CAD build for the part. Positions are in the model's coordinates, mm. Give positions to 0.01 mm unless a question says otherwise; leave off trailing zeros. Order: outer loops, then holes, each group sorted by start corner. A loop starts at its lowest first (then second) coordinate and runs counter-clockwise, first axis right, second up. Notation, with made-up numbers: (67.5, 81.5) -> (105.5, 81.5) arc R35 ccw to (105.5, 120.5) -> close; hole circle Ø3 at (85, 3.5). An arc over 180 degrees is marked (long way). Use one line per item in the form item = value. Start each with the question number.
1) Drop flat-ended pins along their axis: P1, Ø2, axis at y = 2, z = -4.5, coming from the +X side; P2, Ø1.5, axis at y = 8.5, z = 3, coming from the +X side; P3, Ø1.5, axis at x = 2, z = 7.5, coming from the -Y side. Give the stop position or say it passes through.
2) Cut at A-A, the plane x = 1. Give the cut face in (y, z), and give its area (3 significant figures).
3) Probe line 1 (X direction, y = -8.25, z = -1); line 2 (Y direction, x = 2.5, z = -7); line 3 (Y direction, x = 2, z = 4.75). List the from-to ranges inside material, lowest first.
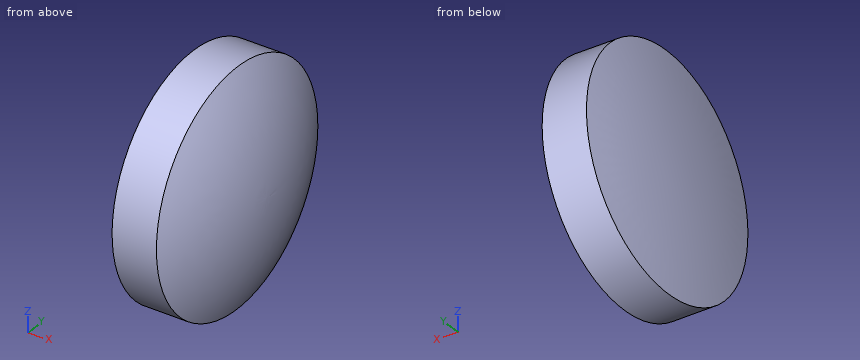
from build123d import *

# Parameters (mm, degrees)
F0_R     = 13.25
F1_DEPTH = 5


with BuildPart() as f1:
    # F0 (on Right) → F1 (new body)
    with BuildSketch(Plane.YZ):
        Circle(F0_R)
    extrude(amount=F1_DEPTH)

    # F2 (on Top) → F4 (revolve)
    with BuildSketch(Plane.XY):
        with BuildLine():
            ThreePointArc((8.325502, 0), (7.481431, 6.830473), (5, 13.25))
            Line((5, 13.25), (5, 0))
            Line((5, 0), (8.325502, 0))
        make_face()
    revolve(axis=Axis((5.30408, 0, 0), (1, 0, 0)))

    # F5 (on Front) → F6 (revolve)
    with BuildSketch(Plane.XZ):
        with BuildLine():
            Line((-1.236098, 0), (0, 0))
            Line((0, 0), (0, 13.25))
            ThreePointArc((0, 13.25), (-0.926404, 6.653767), (-1.236098, 0))
        make_face()
    revolve(axis=Axis((-0.618049, 0, 0), (-1, 0, 0)))


solid = f1.part
Result:
q1.P1 = 8.05
q1.P2 = 7.08
q1.P3 = -11.4
q2.outline = circle Ø26.5 at (0, 0)
q2.area = 552 mm²
q3.line_1 = -0.75 to 7.07
q3.line_2 = -11.25 to 11.25
q3.line_3 = -12.37 to 12.37
